Geometry: final body of the model. Coordinates: model frame, mm. Give positions to 0.01 mm unless a question says otherwise; leave off trailing zeros. Loops run counter-clockwise (first coordinate to the right, second up) from the corner with the lowest first, then second, coordinate; pieces in that order, holes last. Notation, with made-up numbers: (-32, 11) - (-8, 11) arc R21 ccw to (-8, 27) - close; hole circle Ø7 at (0, -38.5). An arc over 180 degrees is marked (long way). Answer in a Markdown table with one row per item.
from build123d import *

# Parameters (mm, degrees)
ESQUISSE1_W              = 300
ESQUISSE1_H              = 300
BOSS_EXTRU_1_DEPTH       = 5
ESQUISSE4_W              = 5
ESQUISSE4_H              = 70.2
ENL_V_MAT_EXTRU_3_DEPTH  = 4.2
ESQUISSE7_R              = 2.1
ENL_V_MAT_EXTRU_6_DEPTH  = 213.190951739
ESQUISSE8_W              = 30
ESQUISSE8_H              = 40
ENL_V_MAT_EXTRU_7_DEPTH  = 213.190951739
ESQUISSE9_R              = 4
ENL_V_MAT_EXTRU_8_DEPTH  = 213.190951739
ESQUISSE10_R             = 2.1
ENL_V_MAT_EXTRU_9_DEPTH  = 213.190951739
ESQUISSE11_W             = 15
ESQUISSE11_H             = 15
ENL_V_MAT_EXTRU_10_DEPTH = 213.190951739
ENL_V_MAT_EXTRU_11_DEPTH = 213.190951739
ESQUISSE13_R             = 2.1
ENL_V_MAT_EXTRU_12_DEPTH = 213.190951739


with BuildPart() as part:
    # Esquisse1 → Boss.-Extru.1 (new body)
    with BuildSketch(Plane.XY):
        Rectangle(ESQUISSE1_W, ESQUISSE1_H)
    extrude(amount=BOSS_EXTRU_1_DEPTH)

    # Esquisse4 → Enlèv. mat.-Extru.3 (cut)
    with BuildSketch(Plane.ZY.offset(150)):
        with Locations((2.5, 114.9)):
            Rectangle(ESQUISSE4_W, ESQUISSE4_H)
        with Locations((2.5, -114.9)):
            Rectangle(ESQUISSE4_W, ESQUISSE4_H)
    extrude(amount=-ENL_V_MAT_EXTRU_3_DEPTH, mode=Mode.SUBTRACT)

    # Esquisse7 → Enlèv. mat.-Extru.6 (cut, through all)
    with BuildSketch(Plane.XY.offset(5)):
        with Locations((135, -135)):
            Circle(ESQUISSE7_R)
        with Locations(Location((135, 135, 0), (0, 0, 180))):
            Circle(ESQUISSE7_R)
    extrude(amount=-ENL_V_MAT_EXTRU_6_DEPTH, mode=Mode.SUBTRACT)

    # Esquisse8 → Enlèv. mat.-Extru.7 (cut, through all)
    with BuildSketch(Plane(origin=(0, 0, 0), x_dir=(-1, 0, 0), z_dir=(0, 0, -1))):
        with Locations((14.345984425, 0)):
            Rectangle(ESQUISSE8_W, ESQUISSE8_H)
    extrude(amount=-ENL_V_MAT_EXTRU_7_DEPTH, mode=Mode.SUBTRACT)

    # Esquisse9 → Enlèv. mat.-Extru.8 (cut, through all)
    with BuildSketch(Plane(origin=(0, 0, 0), x_dir=(-1, 0, 0), z_dir=(0, 0, -1))):
        with Locations((136, 57.5)):
            Circle(ESQUISSE9_R)
        with Locations(Location((136, -57.5, 0), (0, 0, 180))):
            Circle(ESQUISSE9_R)
    extrude(amount=-ENL_V_MAT_EXTRU_8_DEPTH, mode=Mode.SUBTRACT)

    # Esquisse10 → Enlèv. mat.-Extru.9 (cut, through all)
    with BuildSketch(Plane(origin=(0, 0, 0), x_dir=(-1, 0, 0), z_dir=(0, 0, -1))):
        with Locations((-85, 119.5)):
            Circle(ESQUISSE10_R)
        with Locations(Location((-85, -119.5, 0), (0, 0, 180))):
            Circle(ESQUISSE10_R)
    extrude(amount=-ENL_V_MAT_EXTRU_9_DEPTH, mode=Mode.SUBTRACT)

    # Esquisse11 → Enlèv. mat.-Extru.10 (cut, through all)
    with BuildSketch(Plane(origin=(0, 0, 0), x_dir=(-1, 0, 0), z_dir=(0, 0, -1))):
        with Locations((14.345984425, 119.5)):
            Rectangle(ESQUISSE11_W, ESQUISSE11_H)
        with Locations((14.345984425, -119.5)):
            Rectangle(ESQUISSE11_W, ESQUISSE11_H)
    extrude(amount=-ENL_V_MAT_EXTRU_10_DEPTH, mode=Mode.SUBTRACT)

    # Esquisse12 → Enlèv. mat.-Extru.11 (cut, through all)
    with BuildSketch(Plane(origin=(0, 0, 0), x_dir=(-1, 0, 0), z_dir=(0, 0, -1))):
        Polygon((145.8, -115), (145.8, -117.1), (139, -117.1), (139, -118.5), (135.8, -118.5), (135.8, -117.1), (128.8, -117.1), (128.8, -112.9), (135.8, -112.9), (135.8, -111.5), (139, -111.5), (139, -112.9), (145.8, -112.9), align=None)
        Polygon((145.8, 115), (145.8, 112.9), (139, 112.9), (139, 111.5), (135.8, 111.5), (135.8, 112.9), (128.8, 112.9), (128.8, 117.1), (135.8, 117.1), (135.8, 118.5), (139, 118.5), (139, 117.1), (145.8, 117.1), align=None)
    extrude(amount=-ENL_V_MAT_EXTRU_11_DEPTH, mode=Mode.SUBTRACT)

    # Esquisse13 → Enlèv. mat.-Extru.12 (cut, through all)
    with BuildSketch(Plane(origin=(0, 0, 0), x_dir=(-1, 0, 0), z_dir=(0, 0, -1))):
        with Locations((132.95, 25.85)):
            Circle(ESQUISSE13_R)
        with Locations(Location((132.95, -25.85, 0), (0, 0, 180))):
            Circle(ESQUISSE13_R)
    extrude(amount=-ENL_V_MAT_EXTRU_12_DEPTH, mode=Mode.SUBTRACT)


solid = part.part
Q1. Draft query along Y for faces 1 (the flat face through (-2, 35, 5)), 2 (the cylindrical face through (-135.133, 53.595, 2.465)). Return one class per face: pulls with the +Y half, pulls with the -Y half, needs draft (parallel to the pull), parting line crosses it, or undercut.
Check values:
| item | result |
|---|---|
| face 1 | needs draft |
| face 2 | undercut |
Q2. Cut plane A-A (x = -12.5). Output: boundary loops of the cut face in (y, z).
Check values:
| item | result |
|---|---|
| outline | (-150, 0) - (-127, 0) - (-127, 5) - (-150, 5) - close; (-112, 0) - (-20, 0) - (-20, 5) - (-112, 5) - close; (20, 0) - (112, 0) - (112, 5) - (20, 5) - close; (127, 0) - (150, 0) - (150, 5) - (127, 5) - close |
Q3. Cut plane C-C (z = 2.15). Give the number of separate pieces and of enclosed holes in the cut face, and give its area (3 significant figures).
Check values:
| item | result |
|---|---|
| separate pieces | 1 |
| enclosed holes | 11 |
| area | 87,400 mm² |
Q4. First-contact query: pin 1 (1.5 mm diameter, centred on y = -112.5, z = 2.5, fed in from -X). Flat tip, straight axial feed; report the tip coordinate or a pass-through.
Check values:
| item | result |
|---|---|
| pin 1 | x = -145.8 |
Q5. Material intervals for line 1 along Y through (x, z) = (85, 2.8); line 2 along Y through (x, z) = (-136, 2.4); line 3 along X through (y, z) = (-25.85, 1.95), sorted ascending.
Check values:
| item | result |
|---|---|
| line 1 | -150 to -121.6, -117.4 to 117.4, 121.6 to 150 |
| line 2 | -150 to -118.5, -111.5 to -61.5, -53.5 to 53.5, 61.5 to 111.5, 118.5 to 150 |
| line 3 | -150 to -135.05, -130.85 to 150 |
Q6. Cut plane B-B (y = -57.5). Output: boundary loops of the cut face in (x, z), and give its area (3 significant figures).
Check values:
| item | result |
|---|---|
| outline | (-150, 0) - (-140, 0) - (-140, 5) - (-150, 5) - close; (-132, 0) - (150, 0) - (150, 5) - (-132, 5) - close |
| area | 1,460 mm² |
